The listing builds one solid part. Answer for the finished solid, in the listing's coordinates (mm). Face numbers are marked on the shaded views. A direction names the side the tool comes from. Give positions to 0.01 mm unless a question says otherwise; leave off trailing zeros. Write each loop counter-clockwise with the first axis right and the second up, starting at its lowest first coordinate (ties: lowest second). Pieces come first, ordered by that corner, then holes.
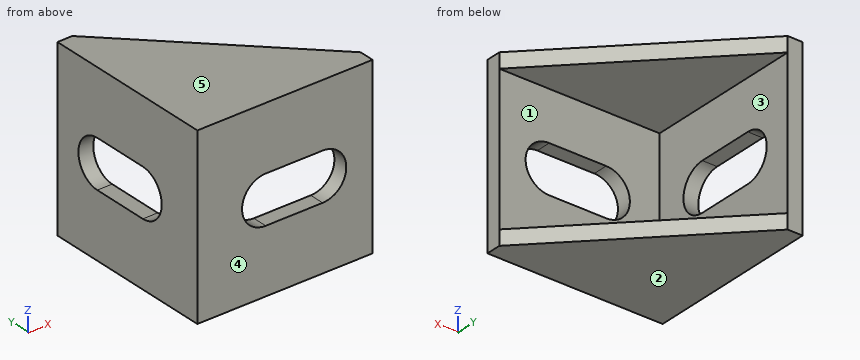
```python
from build123d import *

# Parameters (mm, degrees)
SKICA1_W                 = 20
SKICA1_H                 = 20
P_IDAT_VYSUNUT_M1_DEPTH  = 1.7
SKICA2_W                 = 1.7
SKICA2_H                 = 20
P_IDAT_VYSUNUT_M2_DEPTH  = 18.3
ODEBRAT_VYSUNUT_M1_DEPTH = 1.7
SKICA4_W                 = 1.7
SKICA4_H                 = 18.3
P_IDAT_VYSUNUT_M3_DEPTH  = 18.3
ZKOSEN_1_SIZE            = 18.3


with BuildPart() as part:
    # Skica1 → Přidat vysunutím1 (new body)
    with BuildSketch(Plane(origin=(0, 0, 0), x_dir=(1, 0, 0), z_dir=(0, 1, 0))):
        Rectangle(SKICA1_W, SKICA1_H)
        with BuildLine():
            Line((-2.2, 2.7), (4.3, 2.7))
            ThreePointArc((4.3, 2.7), (7, 0), (4.3, -2.7))
            Line((4.3, -2.7), (-2.2, -2.7))
            ThreePointArc((-2.2, -2.7), (-4.9, 0), (-2.2, 2.7))
        make_face(mode=Mode.SUBTRACT)
    extrude(amount=P_IDAT_VYSUNUT_M1_DEPTH)

    # Skica2 → Přidat vysunutím2 (add)
    with BuildSketch(Plane(origin=(0, 1.7, 0), x_dir=(1, 0, 0), z_dir=(0, 1, 0))):
        with Locations((-9.15, 0)):
            Rectangle(SKICA2_W, SKICA2_H)
    extrude(amount=P_IDAT_VYSUNUT_M2_DEPTH)

    # Skica3 → Odebrat vysunutím1 (cut)
    with BuildSketch(Plane(origin=(-8.3, 0, 0), x_dir=(0, 0, -1), z_dir=(1, 0, 0))):
        with BuildLine():
            Line((2.7, 14.3), (2.7, 7.8))
            ThreePointArc((2.7, 7.8), (0, 5.1), (-2.7, 7.8))
            Line((-2.7, 7.8), (-2.7, 14.3))
            ThreePointArc((-2.7, 14.3), (0, 17), (2.7, 14.3))
        make_face()
    extrude(amount=-ODEBRAT_VYSUNUT_M1_DEPTH, mode=Mode.SUBTRACT)

    # Skica4 → Přidat vysunutím3 (add)
    with BuildSketch(Plane(origin=(-8.3, 0, 0), x_dir=(0, 0, -1), z_dir=(1, 0, 0))):
        with Locations((-9.15, 10.85)):
            Rectangle(SKICA4_W, SKICA4_H)
        with Locations((9.15, 10.85)):
            Rectangle(SKICA4_W, SKICA4_H)
    extrude(amount=P_IDAT_VYSUNUT_M3_DEPTH)

    # Zkosení1
    zkosen_1_edges = [part.edges().sort_by_distance(p)[0] for p in [
        (10, 20, -9.15),
        (10, 20, 9.15),
    ]]
    chamfer(zkosen_1_edges, length=ZKOSEN_1_SIZE)


solid = part.part
```
Item 1: A cutting plane is placed at A-A, the plane x = 0.5. Give the vertices of the cut face in (y, z).
Conclusion:
outline: (0, -10) - (11.2, -10) - (11.2, -8.3) - (1.7, -8.3) - (1.7, -2.7) - (0, -2.7) - close; (0, 2.7) - (1.7, 2.7) - (1.7, 8.3) - (11.2, 8.3) - (11.2, 10) - (0, 10) - close
Item 2: A cutting plane is placed at D-D, the plane y = 3.5. Give the vertices of the cut face in (x, z).
Conclusion:
outline: (-10, -10) - (8.2, -10) - (8.2, -8.3) - (-8.3, -8.3) - (-8.3, 8.3) - (8.2, 8.3) - (8.2, 10) - (-10, 10) - close
Item 3: Each of these flat-tipped pins is pushed along its axis until it touches: P1, Ø5, axis at y = 14, z = 2, coming from the -X side; P2, Ø5, axis at x = 3.5, z = 2.5, coming from the +Y side; P3, Ø1, axis at x = 4.5, z = 2, coming from the -Y side. Where does it stop, or does it pass through?
Conclusion:
P1: stops at x = -10
P2: stops at y = 1.7
P3: passes through
Item 4: Which of the six approach directions +Z, -Z, +X, -X, +Y, -Y give full straight-line access (tool end or side, diameter ignored) to the marked faces 1 and 2?
Conclusion:
face 1: +X, +Y
face 2: -Z, +X, -X, +Y, -Y
Item 5: Determine the mould class of the marked faces 3, 4 and 5 for opening direction Z: pulls with the +Z half, pulls with the -Z half, needs draft (parallel to the pull), parting line crosses it, or undercut.
Conclusion:
face 3: undercut
face 4: needs draft
face 5: pulls with the +Z half
Item 6: Consider probe 1 along Z at (x, y) = (-7.5, 11.5); probe 2 along X at (y, z) = (11.5, 5.75); probe 3 along Y at (x, z) = (8.25, 7.25). Determine where each line is inside the solid, lowest interval first.
Conclusion:
probe 1: z = -10 to -8.3, 8.3 to 10
probe 2: x = -10 to -8.3
probe 3: y = 0 to 1.7
Item 7: A cutting plane is placed at B-B, the plane y = 11.75. Give the vertices of the cut face in (x, z), plus the area to 3 significant figures.
Conclusion:
outline: (-10, -10) - (-0.05, -10) - (-0.05, -8.3) - (-8.3, -8.3) - (-8.3, -2.7) - (-10, -2.7) - close; (-10, 2.7) - (-8.3, 2.7) - (-8.3, 8.3) - (-0.05, 8.3) - (-0.05, 10) - (-10, 10) - close
area: 52.9 mm2
Item 8: A cutting plane is placed at C-C, the plane z = 0. Give the vertices of the cut face in (x, y), plus the area to 4 significant figures.
Conclusion:
outline: (-10, 0) - (-4.9, 0) - (-4.9, 1.7) - (-8.3, 1.7) - (-8.3, 5.1) - (-10, 5.1) - close; (-10, 17) - (-8.3, 17) - (-8.3, 20) - (-10, 20) - close; (7, 0) - (10, 0) - (10, 1.7) - (7, 1.7) - close
area: 24.65 mm2
